Geometry check sheet. Reference: the model listing, model coordinates, mm. Face numbers are marked on the shaded views. A direction names the side the tool comes from. Round coordinates to 2 decimals unless told otherwise and drop trailing zeros. Loops run counter-clockwise (first coordinate to the right, second up) from the corner with the lowest first, then second, coordinate; pieces in that order, holes last. Notation, with made-up numbers: M 58,73 L 65,73 A21 cw 65,92 Z; hole C 69,-10 d10. An arc over 180 degrees is marked long. Write item = value, one per line.
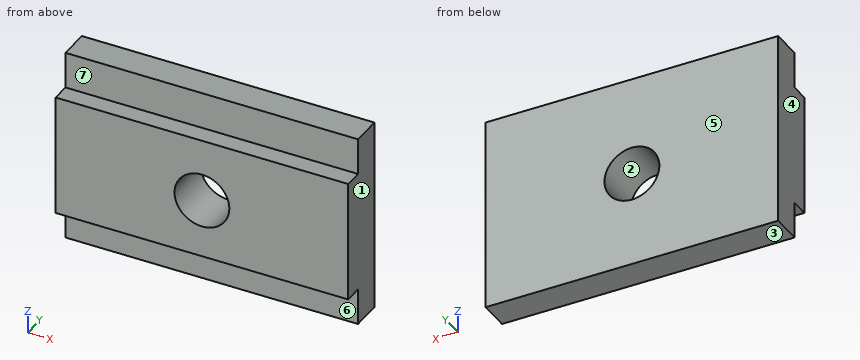
from build123d import *

# Parameters (mm, degrees)
F0_R     = 14.2875
F0_W     = 152.4
F0_H     = 19.05
F1_DEPTH = 15.875
F2_DEPTH = 25.4


with BuildPart() as f1:
    # F0 (on Front) → F1 (new body)
    with BuildSketch(Plane.XZ):
        Polygon((-9.553027, 51.909848), (-85.753027, 51.909848), (-85.753027, 32.859848), (66.646973, 32.859848), (66.646973, 51.909848), align=None)
        Polygon((66.646973, 32.859848), (-85.753027, 32.859848), (-85.753027, -30.640152), (66.646973, -30.640152), (66.646973, 0), align=None)
        with Locations((-9.553027, 0)):
            Circle(F0_R, mode=Mode.SUBTRACT)
        with Locations((-9.553027, -40.165152)):
            Rectangle(F0_W, F0_H)
    extrude(amount=F1_DEPTH)

    # F0 (on Front) → F2 (join)
    with BuildSketch(Plane.XZ):
        Polygon((66.646973, 32.859848), (-85.753027, 32.859848), (-85.753027, -30.640152), (66.646973, -30.640152), (66.646973, 0), align=None)
        with Locations((-9.553027, 0)):
            Circle(F0_R, mode=Mode.SUBTRACT)
    extrude(amount=F2_DEPTH)


solid = f1.part
(1) Depth check by flat-ended pin: pin 1 Ø15 at (x, z) = (9, -38.5) entering from -Y (3 decimals); pin 2 Ø5 at (x, y) = (-22.5, -19.5) entering from -Z; pin 3 Ø5 at (x, y) = (13.5, -22.5) entering from +Z; pin 4 Ø23 at (x, z) = (-9.55, 0) entering from +Y. Enter the tip coordinate at first touch or a pass-through.
Result set:
pin_1 = -15.875
pin_2 = -30.64
pin_3 = 32.86
pin_4 = through
(2) Sectioned sample at B-B on y = -17.5. Record the cut outline in (x, z) (1 decimal).
Result set:
outline = M -85.8,-30.6 L 66.6,-30.6 L 66.6,32.9 L -85.8,32.9 Z; hole C -9.6,0 d28.6
(3) Sectioned sample at D-D on z = -43. Record the cut outline in (x, y) (3 decimals), then the cut area to 3 significant figures.
Result set:
outline = M -85.753,-15.875 L 66.647,-15.875 L 66.647,0 L -85.753,0 Z
area = 2,420 mm2
(4) Release check for a two-part mould opening along X. For the marked faces 1, 2, 3 and 4 record: released by +X, released by -X, zero draft, split by the parting line, or undercut.
Result set:
face_1 = released by +X
face_2 = undercut
face_3 = zero draft
face_4 = released by -X
(5) Tool access check on the marked faces 5, 6 and 7. Record the directions out of +Z, -Z, +X, -X, +Y, -Y that give a thin tool (end or side, any length) a straight path to the whole face; none if there is none.
Result set:
face_5 = +Z, -Z, +X, -X, +Y
face_6 = -Z, +X, -X, -Y
face_7 = +Z, +X, -X, -Y
(6) Sectioned sample at A-A on z = 0. Record the cut outline in (x, y), then the cut area to 3 significant figures.
Result set:
outline = M -85.75,-25.4 L -23.84,-25.4 L -23.84,0 L -85.75,0 Z; M 4.73,-25.4 L 66.65,-25.4 L 66.65,0 L 4.73,0 Z
area = 3,150 mm2
(7) Material ranges on line 1 along Z through (x, y) = (-49, -21.5); line 2 along Y through (x, z) = (0.5, 48) (3 decimals); line 3 along X through (y, z) = (-4.75, -13), recorded low to high. Write a range as from..to.
Result set:
line_1 = -30.64..32.86
line_2 = -15.875..0
line_3 = -85.75..-15.48, -3.63..66.65
(8) Sectioned sample at C-C on x = 51. Record the cut outline in (y, z) (3 decimals).
Result set:
outline = M -25.4,-30.64 L -15.875,-30.64 L -15.875,-49.69 L 0,-49.69 L 0,51.91 L -15.875,51.91 L -15.875,32.86 L -25.4,32.86 Z
